Autodesk Inventor part; units mm, degrees
ref_plane "YZ Plane" through (0, 0, 0) normal (1, 0, 0) x (0, 1, 0)
ref_plane "XZ Plane" through (0, 0, 0) normal (0, 1, 0) x (-1, 0, 0)
ref_plane "XY Plane" through (0, 0, 0) normal (0, 0, 1) x (1, 0, 0)
sketch "Sketch1" plane through (0, 0, 0) normal (1, 0, 0) x (0, 1, 0)
  line L0 (16, 0) -> (16, 5)
  line L1 (16, 5) -> (15, 5)
  line L2 (15, 5) -> (15, 7)
  line L3 (15, 7) -> (16, 7)
  line L4 (16, 7) -> (16, 14)
  line L5 (16, 14) -> (14, 14)
  line L6 (14, 14) -> (14, 17)
  line L7 (18, 0) -> (18, 17)
  line L8 (18, 17) -> (14, 17)
  line L9 (16, 0) -> (18, 0)
  line L10 (0, 0) -> (0, 15) construction
  dimension "d0" = 5
  dimension "d1" = 16
  dimension "d2" = 1
  dimension "d3" = 2
  dimension "d4" = 7
  dimension "d8" = 14
  dimension "d9" = 3
  dimension "d10" = 18
revolve "Revolution1" add sketch "Sketch1" angle 360 about axis through (0, 0, 0) along (0, 0, 1)
thread "Thread1"
fillet "Fillet1" radius 2 1 edges at (0, -18, 17)
properties part number "201-02" material "PC/ABS Plastic"
CAD build for the part. Positions are in the model's coordinates, mm. A direction names the side the tool comes from. Coordinates: 2 decimals unless noted, no trailing zeros. Write each loop counter-clockwise with the first axis right and the second up, starting at its lowest first coordinate (ties: lowest second). Pieces come first, ordered by that corner, then holes. Notation, with made-up numbers: (80.5, 71) - (85.5, 71) arc R24 ccw to (85.5, 104) - close; hole circle Ø1 at (79.5, 72). An arc over 180 degrees is marked (long way). Use a Markdown table: item, result. Add a question column.
Item 1: Band-saw the part on A-A, the plane x = 0. Give the cut face in (y, z), and give its area (3 significant figures).
Item 2: Flat gauge pins, fed straight in: pin 1 (10 mm diameter, centred on y = 3.5, z = 3, fed in from -X); pin 2 (5 mm diameter, centred on y = -11.5, z = 3, fed in from +X); pin 3 (1 mm diameter, centred on y = -5, z = 11, fed in from +X). Where does each tip first touch, or does it go through?
Item 3: 3-axis set-ups, long thin cutter, end or side, ignore diameter. For faces 4 (the face through (14.15, -0.07, 17)), 5 (the face through (15.62, -3.47, 2.54)), 6 (the face through (15.62, -3.47, 10.55)): which of +Z, -Z, +X, -X, +Y, -Y reach the whole face in a straight line?
Item 4: Mould opens along X. For faces 1 (the face through (11, -12, 0)), 2 (the face through (5.362, 12.932, 15.521)), 3 (the face through (-17.847, -2.343, 7.605)) say: pulls with the +X half, pulls with the -X half, needs draft (parallel to the pull), parting line crosses it, or undercut.
Item 5: Band-saw the part on D-D, the plane z = 15.5. Give the cut face in (x, y).
Item 6: Drill centre lines: L1, parallel to Z at x = -15, y = -2; L2, parallel to X at y = 0, z = 2.4; L3, parallel to Y at x = 5, z = 5.75. Where is each one in solid material? Low to high. Write a range as from..to.
Item 7: Band-saw the part on C-C, the plane z = 13.5. Give the cut face in (x, y), and give its area (3 significant figures).
Numbers:
| question | item | result |
|---|---|---|
| 1 | outline | (-18, 0) - (-16, 0) - (-16, 5) - (-15, 5) - (-15, 7) - (-16, 7) - (-16, 14) - (-14, 14) - (-14, 17) - (-16, 17) arc R2 ccw to (-18, 15) - close; (14, 14) - (16, 14) - (16, 7) - (15, 7) - (15, 5) - (16, 5) - (16, 0) - (18, 0) - (18, 15) arc R2 ccw to (16, 17) - (14, 17) - close |
| 1 | area | 82.3 mm2 |
| 2 | pin 1 | x = -18 |
| 2 | pin 2 | x = 15.59 |
| 2 | pin 3 | x = 17.43 |
| 3 | face 4 | +Z, +X, -X, +Y, -Y |
| 3 | face 5 | -Z |
| 3 | face 6 | none |
| 4 | face 1 | needs draft |
| 4 | face 2 | undercut |
| 4 | face 3 | parting line crosses it |
| 5 | outline | circle Ø35.87 at (0, 0); hole circle Ø28 at (0, 0) |
| 6 | L1 | 5..7, 14..17 |
| 6 | L2 | -18..-16, 16..18 |
| 6 | L3 | -17.29..-14.14, 14.14..17.29 |
| 7 | outline | circle Ø36 at (0, 0); hole circle Ø32 at (0, 0) |
| 7 | area | 214 mm2 |
